Could you check a few things on this model? Use its own coordinates, in mm. Face numbers are marked on the shaded views. A direction names the side the tool comes from. Give positions to 0.01 mm unless a question says otherwise; leave off trailing zeros. Loops run counter-clockwise (first coordinate to the right, second up) from the corner with the lowest first, then second, coordinate; pieces in that order, holes last. Notation, with made-up numbers: (-20, 5.25) - (-9, 5.25) arc R35 ccw to (-9, 38.25) - close; hole circle Ø9 at (-18, -13.75). An arc over 180 degrees is marked (long way). Write each question's results on one line, items separated by ' | '. Start each with the question number.
(1) On a 3-axis mill with a long thin cutter (end or side, diameter ignored), from which of +Z, -Z, +X, -X, +Y, -Y can I reach the whole of each face in a straight line? I mean the marked faces 1 and 2. Say none if no direction works.
(2) I need wall thicknesses on line 1 (Z direction, x = 644.5, y = 210); line 2 (Y direction, x = 665, z = 23.5); line 3 (Z direction, x = 739, y = 214.5). Which ranges of each line are inside material? Lowest first, please.
(3) Suppose I cut it at C-C (z = 20.5). Please give me the cut outline in (x, y).
(4) Suppose I cut it at A-A (y = 215). Please give me the cut outline in (x, z).
(5) If we mould it in two halves opening along X, with no side actions, what happens to the marked faces 3, 4 and 5? For each: released by +X, released by -X, zero draft, split by the parting line, or undercut.
(6) For pin 1 (10 mm diameter, centred on x = 686.5, y = 191, fed in from +Z); pin 2 (12.5 mm diameter, centred on x = 693, z = 29.5, fed in from -Y); pin 3 (7 mm diameter, centred on x = 640.5, y = 190.5, fed in from +Z), each with a flat end and sliding along its axis, tell me the tip position at first contact or that it passes through.
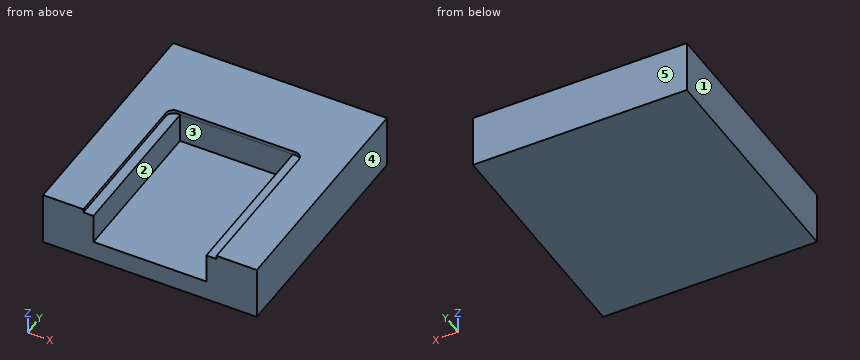
from build123d import *

# Parameters (mm, degrees)
SKETCH151_W     = 180
SKETCH151_H     = 200
PAD010_DEPTH    = 45
SKETCH152_W     = 112
SKETCH152_H     = 133
POCKET030_DEPTH = 3
SKETCH153_W     = 95
SKETCH153_H     = 134
POCKET031_DEPTH = 25
FILLET009_R     = 6.35


with BuildPart() as part:
    # Sketch151 → Pad010 (new body)
    with BuildSketch(Plane.XY):
        with Locations((690, 200)):
            Rectangle(SKETCH151_W, SKETCH151_H)
    extrude(amount=PAD010_DEPTH)

    # Sketch152 (on Face6 of Pad010) → Pocket030 (cut)
    with BuildSketch(Plane.XY.offset(45)):
        with Locations((690, 166.5)):
            Rectangle(SKETCH152_W, SKETCH152_H)
    extrude(amount=-POCKET030_DEPTH, mode=Mode.SUBTRACT)

    # Sketch153 (on Face6 of Pocket030) → Pocket031 (cut)
    with BuildSketch(Plane.XY.offset(42)):
        with Locations((690.00001, 166.000003)):
            Rectangle(SKETCH153_W, SKETCH153_H)
    extrude(amount=-POCKET031_DEPTH, mode=Mode.SUBTRACT)

    # Fillet009
    fillet009_edges = [part.edges().sort_by_distance(p)[0] for p in [
        (634, 233, 43.5),
        (746, 233, 43.5),
    ]]
    fillet(fillet009_edges, radius=FILLET009_R)


solid = part.part
Output values:
1) face 1: +Z, -Z, -X, +Y, -Y | face 2: +Z, -Y
2) line 1: 0 to 17 | line 2: 233 to 300 | line 3: 0 to 42
3) outline: (600, 100) - (642.5, 100) - (642.5, 233) - (737.5, 233) - (737.5, 100) - (780, 100) - (780, 300) - (600, 300) - close
4) outline: (600, 0) - (780, 0) - (780, 45) - (746, 45) - (746, 42) - (737.5, 42) - (737.5, 17) - (642.5, 17) - (642.5, 42) - (634, 42) - (634, 45) - (600, 45) - close
5) face 3: undercut | face 4: released by +X | face 5: zero draft
6) pin 1: z = 17 | pin 2: y = 233 | pin 3: z = 42
